Geometry check sheet. Reference: the model listing, model coordinates, mm. A direction names the side the tool comes from. Coordinates: 2 decimals unless noted, no trailing zeros. Write each loop counter-clockwise with the first axis right and the second up, starting at its lowest first coordinate (ties: lowest second). Pieces come first, ordered by that corner, then holes. Notation, with made-up numbers: (-18.75, 81) -> (26.25, 81) arc R16 ccw to (26.25, 98) -> close; hole circle Ø8 at (-4.75, 71). An arc over 180 degrees is marked (long way). One line per question, with ' | ' between items.
from build123d import *

# Parameters (mm, degrees)
F2_R     = 1
F3_DEPTH = 1.5
F4_SIZE  = 0.2
F5_R     = 0.4
F6_DEPTH = 0.4
F9_COUNT = 4


with BuildPart() as f1:
    # F0 (on Top) → F1 (revolve)
    with BuildSketch(Plane.XY):
        with BuildLine():
            Line((-6.5, 0), (0, 0))
            Line((0, 0), (0, 4.5))
            Line((0, 4.5), (-3.7298287009, 4.5))
            ThreePointArc((-3.7298287009, 4.5), (-4.9400816795, 4.0922586874), (-5.6568645201, 3.0352877276))
            Line((-5.6568645201, 3.0352877276), (-6.5, 0))
        make_face()
    revolve(axis=Axis((0, 13.4025972581, 0), (0, 1, 0)))

    # F2 (on face) → F3 (join)
    with BuildSketch(Plane(origin=(0, 4.5, 0), x_dir=(-1, 0, 0), z_dir=(0, 1, 0))):
        Circle(F2_R)
    extrude(amount=F3_DEPTH)

    # F4
    f4_edges = [f1.edges().sort_by_distance(p)[0] for p in [
        (1, 6, 0),
    ]]
    chamfer(f4_edges, length=F4_SIZE)

    # F5 (on face) → F6 (join)
    with BuildSketch(Plane(origin=(0, 4.5, 0), x_dir=(-1, 0, 0), z_dir=(0, 1, 0))):
        with Locations((0, 3.2)):
            Circle(F5_R)
        with Locations((3.2, 0)):
            Circle(F5_R)
        with Locations((0, -3.2)):
            Circle(F5_R)
        with Locations((-3.2, 0)):
            Circle(F5_R)
        with Locations((-2.2627416998, 2.2627416998)):
            Circle(F5_R)
        with Locations((2.2627416998, 2.2627416998)):
            Circle(F5_R)
        with Locations((2.2627416998, -2.2627416998)):
            Circle(F5_R)
        with Locations((-2.2627416998, -2.2627416998)):
            Circle(F5_R)
    extrude(amount=F6_DEPTH)


with BuildPart() as f8:
    # F7 (on Right) → F8 (revolve)
    with BuildSketch(Plane.YZ):
        Polygon((-0.7489218035, 8.783760689), (-1.07009444, 7.6275391974), (6.0141044293, 5.6597061782), (6.3352770658, 6.8159276697), align=None)
    revolve(axis=Axis((0, 4.9801668253, 5.9469110682), (0, 0.9635179096, -0.2676438638)))


with BuildPart() as f9_1:
    # F9: instance of F8
    add(f8.part.rotate(Axis((0, 5.8, 0), (0, 1, 0)), 1 * 360 / F9_COUNT))


with BuildPart() as f9_2:
    # F9: instance of F8
    add(f8.part.rotate(Axis((0, 5.8, 0), (0, 1, 0)), 2 * 360 / F9_COUNT))


with BuildPart() as f9_3:
    # F9: instance of F8
    add(f8.part.rotate(Axis((0, 5.8, 0), (0, 1, 0)), 3 * 360 / F9_COUNT))


with BuildPart() as f1_1:
    add(f1.part)

    # F10: cut F8, F9_1, F9_2, F9_3
    add(f8.part, mode=Mode.SUBTRACT)
    add(f9_1.part, mode=Mode.SUBTRACT)
    add(f9_2.part, mode=Mode.SUBTRACT)
    add(f9_3.part, mode=Mode.SUBTRACT)


solid = f1_1.part
1. Material ranges on line 1 (Y direction, x = 1, z = -3); line 2 (Z direction, x = 1, y = 4); line 3 (X direction, y = 0.5, z = 0), recorded low to high. Write a range as from..to.
Worked answers:
line 1: 0..4.5 | line 2: -4.95..4.95 | line 3: -5.95..5.95
2. Cross-section at C-C on y = 4.25. Record the boundary of the cut face in (x, z).
Worked answers:
outline: circle Ø9.4 at (0, 0)
3. Cross-section at B-B on z = 0. Record the boundary of the cut face in (x, y).
Worked answers:
outline: (-6.08, 0) -> (6.08, 0) -> (4.95, 4.08) arc R2 ccw to (3.73, 4.5) -> (3.6, 4.5) -> (3.6, 4.9) -> (2.8, 4.9) -> (2.8, 4.5) -> (1, 4.5) -> (1, 5.8) -> (0.8, 6) -> (-0.8, 6) -> (-1, 5.8) -> (-1, 4.5) -> (-2.8, 4.5) -> (-2.8, 4.9) -> (-3.6, 4.9) -> (-3.6, 4.5) -> (-3.73, 4.5) arc R2 ccw to (-4.95, 4.08) -> close
4. Go/stop test with flat-tipped pins: P1, Ø1.5, axis at y = 2, z = -0.5, coming from the +X side; P2, Ø0.9, axis at x = -2, z = 2.5, coming from the +Y side; P3, Ø1.5, axis at y = 1, z = -3, coming from the -X side. Record where each tip stops, or that it passes through.
Worked answers:
P1: x = 6.07 | P2: y = 4.9 | P3: x = -5.88
5. Cross-section at A-A on x = 0. Record the boundary of the cut face in (y, z).
Worked answers:
outline: (0, -6.08) -> (4.08, -4.95) arc R2 ccw to (4.5, -3.73) -> (4.5, -3.6) -> (4.9, -3.6) -> (4.9, -2.8) -> (4.5, -2.8) -> (4.5, -1) -> (5.8, -1) -> (6, -0.8) -> (6, 0.8) -> (5.8, 1) -> (4.5, 1) -> (4.5, 2.8) -> (4.9, 2.8) -> (4.9, 3.6) -> (4.5, 3.6) -> (4.5, 3.73) arc R2 ccw to (4.08, 4.95) -> (0, 6.08) -> close
6. Mould release check, pull along X, two halves, no side actions. Record for faces 3 (the face through (0, 0, 0)), 4 (the face through (-0.013, 1.968, -5.538)), 5 (the face through (-4.34, 1.5, 4.26)): released by +X, released by -X, zero draft, split by the parting line, or undercut.
Worked answers:
face 3: zero draft | face 4: undercut | face 5: released by -X
7. Tool access check on faces 1 (the face through (1, 4.5, -1)), 2 (the face through (0, 6, 0)). Record the directions out of +Z, -Z, +X, -X, +Y, -Y that give a thin tool (end or side, any length) a straight path to the whole face; none if there is none.
Worked answers:
face 1: +Y | face 2: +Z, -Z, +X, -X, +Y
